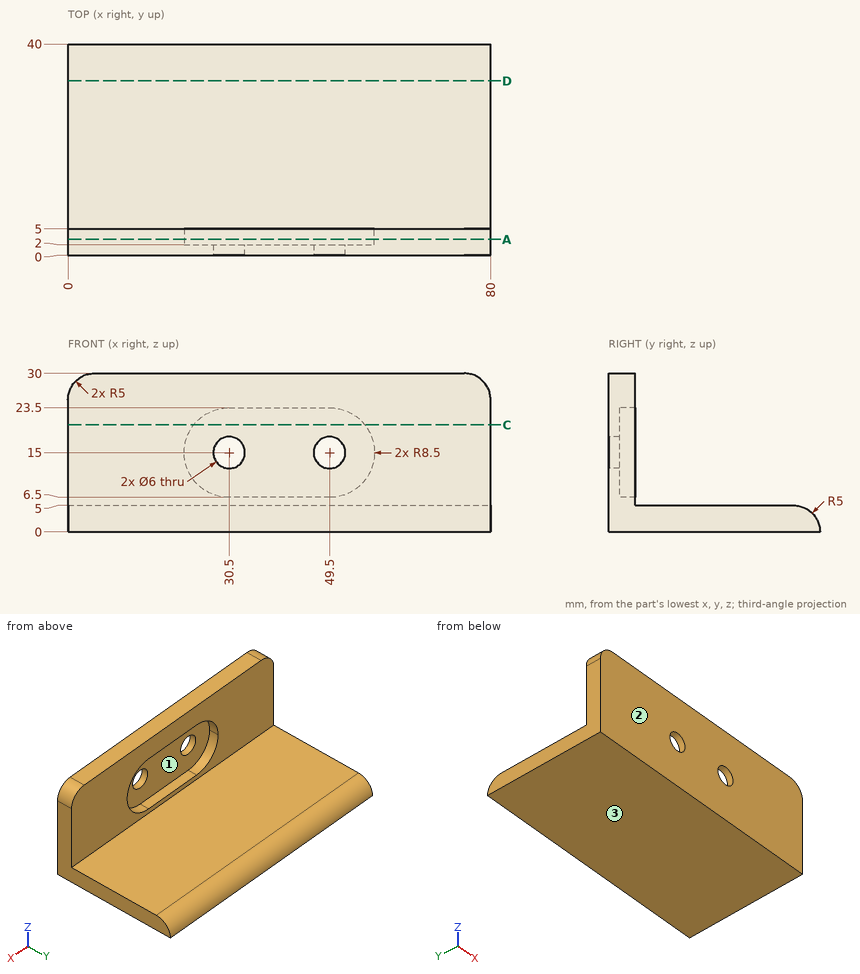
Check sheet for the drawn part. Datum: minimum x, y, z corner. Units: mm. Coordinates: 2 decimals unless noted, no trailing zeros. Loops run counter-clockwise (first coordinate to the right, second up) from the corner with the lowest first, then second, coordinate; pieces in that order, holes last. Notation, with made-up numbers: (21.5, -32.75) -> (57.5, -32.75) arc R11 cw to (57.5, -15.75) -> close; hole circle Ø9 at (49.5, 55.5). An arc over 180 degrees is marked (long way). Answer in a Markdown table with one row per item.
1. Material ranges on line 1 along Z through (x, y) = (49.5, 1.35); line 2 along Z through (x, y) = (44, 4); line 3 along Z through (x, y) = (59.5, 19), recorded low to high. Write a range as [from, to].
Check values:
| item | result |
|---|---|
| line 1 | z = [0, 12], [18, 30] |
| line 2 | z = [0, 6.5], [23.5, 30] |
| line 3 | z = [0, 5] |
2. Sectioned sample at A-A, the plane y = 3. Record the boundary of the cut face in (x, z), then the cut area to 3 significant figures.
Check values:
| item | result |
|---|---|
| outline | (0, 0) -> (80, 0) -> (80, 25) arc R5 ccw to (75, 30) -> (5, 30) arc R5 ccw to (0, 25) -> close; hole (30.5, 6.5) -> (49.5, 6.5) arc R8.5 ccw to (49.5, 23.5) -> (30.5, 23.5) arc R8.5 ccw to start |
| area | 1,840 mm2 |
3. Sectioned sample at D-D, the plane y = 33. Record the boundary of the cut face in (x, z), then the cut area to 3 significant figures.
Check values:
| item | result |
|---|---|
| outline | (0, 0) -> (80, 0) -> (80, 5) -> (0, 5) -> close |
| area | 400 mm2 |
4. Release check for a two-part mould opening along Z. For the marked faces 1, 2 and 3 record: released by +Z, released by -Z, zero draft, split by the parting line, or undercut.
Check values:
| item | result |
|---|---|
| face 1 | undercut |
| face 2 | zero draft |
| face 3 | released by -Z |
5. Go/stop test with flat-tipped pins: pin 1 (3 mm diameter, centred on x = 46, z = 11.5, fed in from +Y); pin 2 (9 mm diameter, centred on x = 27.5, y = 27, fed in from +Z); pin 3 (12 mm diameter, centred on x = 65.5, z = 9.5, fed in from +Y); pin 4 (10 mm diameter, centred on x = 13.5, y = 7.5, fed in from -Z). Record where each tip stops, or that it passes through.
Check values:
| item | result |
|---|---|
| pin 1 | stops at y = 2 |
| pin 2 | stops at z = 5 |
| pin 3 | stops at y = 38.57 |
| pin 4 | stops at z = 0 |
6. Sectioned sample at C-C, the plane z = 20.25. Record the boundary of the cut face in (x, y), then the cut area to 3 significant figures.
Check values:
| item | result |
|---|---|
| outline | (0, 0) -> (80, 0) -> (80, 5) -> (56.18, 5) -> (56.18, 2) -> (23.82, 2) -> (23.82, 5) -> (0, 5) -> close |
| area | 303 mm2 |
